Input: dimensioned drawing with shaded views. Units: mm. Origin: part minimum x, y, z. A direction names the side the tool comes from. Coordinates: 2 decimals unless noted, no trailing zeros.
Item 1: Ray query, line 1 along Y through (x, z) = (12.25, 6.35); line 2 along Y through (x, z) = (3.25, 19.05); line 3 along Z through (x, y) = (66.25, 25.4). Return the intervals inside material, ascending.
Item 2: Section A-A on x = 61. Give the number of separate pieces and of enclosed holes in the cut face, and give its area (3 significant figures).
Item 3: Reachability of the marked faces 1 and 2 from +Z, -Z, +X, -X, +Y, -Y: full face, straight path, thin tool, end or side. Return the list, or none.
Item 4: Contact query for flat-ended pins moving along their axis: P1, Ø4.5, axis at y = 6.35, z = 19.05, coming from the -X side; P2, Ø1.9, axis at y = 44.45, z = 6.35, coming from the +X side; P3, Ø3, axis at y = 6.35, z = 19.05, coming from the -X side. Output: stop coordinate, or through.
Item 5: Pull-direction query (X, two-part tool) for the marked faces 3, 4, 5 and 6; classes: released by +X, released by -X, zero draft, split by the parting line, or undercut.
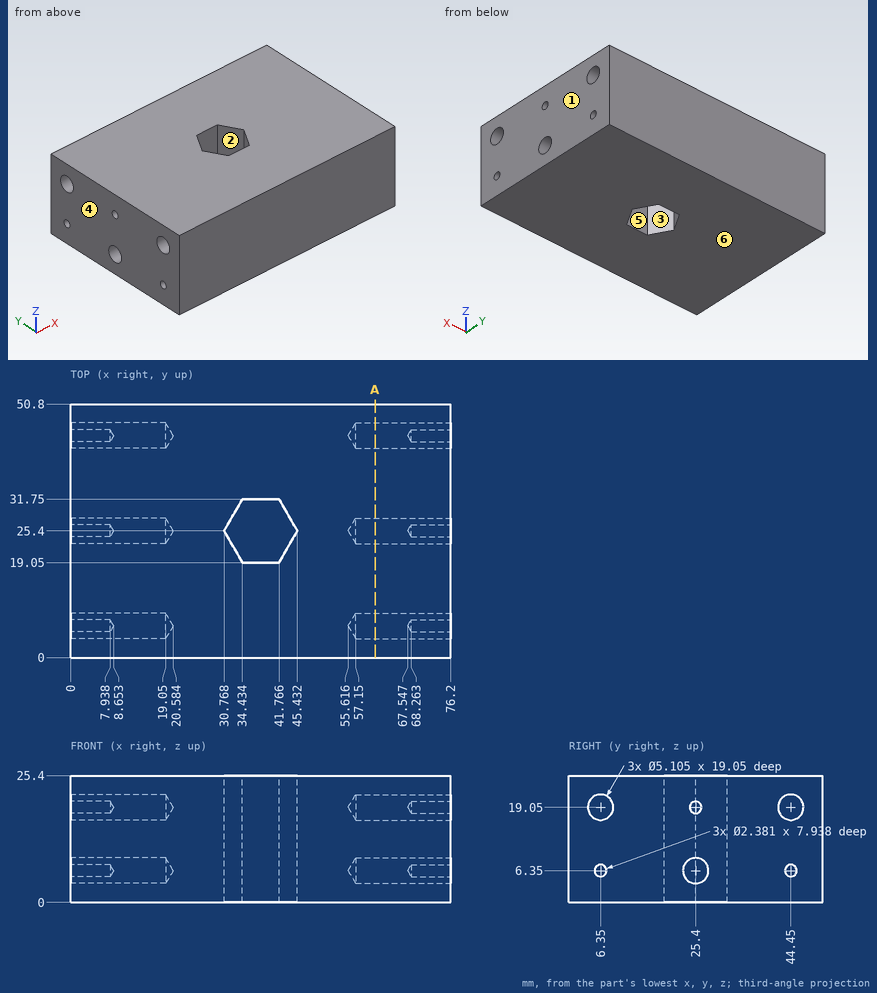
Results found:
1. line 1: y = 0 to 22.85, 27.95 to 50.8
1. line 2: y = 0 to 3.8, 8.9 to 24.21, 26.59 to 41.9, 47 to 50.8
1. line 3: z = 0 to 3.8, 8.9 to 25.4
2. separate pieces: 1
2. enclosed holes: 3
2. area: 1,230 mm2
3. face 1: +Z, -Z, +X, +Y, -Y
3. face 2: +Z, -Z
4. P1: stops at x = 19.23
4. P2: stops at x = 68.12
4. P3: stops at x = 19.68
5. face 3: undercut
5. face 4: released by -X
5. face 5: undercut
5. face 6: zero draft
